Design review of the part built by this model. Coordinates are the model's own, in mm. Face numbers are marked on the shaded views. A direction names the side the tool comes from. Round coordinates to 2 decimals unless told otherwise and drop trailing zeros. Write each loop counter-clockwise with the first axis right and the second up, starting at its lowest first coordinate (ties: lowest second). Pieces come first, ordered by that corner, then holes. Notation, with made-up numbers: (15, -33.75) -> (29, -33.75) arc R24 cw to (29, -9.75) -> close; hole circle Ø5 at (76, 72.5). An arc over 180 degrees is marked (long way). Write item = value, one per line. Start each with the question number.
Item 1: Mouldability with a two-part tool opening along Z and no side actions: class the marked faces 1, 2 and 3 as released by +Z, released by -Z, zero draft, split by the parting line, or undercut.
Item 2: Add section C-C, the plane y = 0.6. State the section outline as (x, z) points.
Item 3: Add section D-D, the plane z = 1.5. State the section outline as (x, y) points.
Item 4: To check wall thickness, follow L1, parallel to Z at x = 3, y = 3.55; L2, parallel to Z at x = -2.25, y = 4; L3, parallel to X at y = 1.8, z = 4. State the ranges of each line that lie inside material, in increasing order.
Item 5: Machinability: for the marked faces 4 and 5, which of the approach directions +Z, -Z, +X, -X, +Y, -Y give a long, thin tool a straight path to every point of the face, cutting with its end or side? Answer none if there is none.
Item 6: Add section A-A, the plane x = 0. State the section outline as (y, z) points.
Item 7: For pin 1 Ø1 at (x, y) = (1.5, 3) entering from +Z; pin 2 Ø2.5 at (x, z) = (0, -4) entering from -Y; pin 3 Ø6 at (x, z) = (0, 4) entering from +Y; pin 4 Ø1 at (x, y) = (-4, 0.5) entering from -Z, all flat-tipped, find the tip position at first contact; note any pin that passes through.
Item 8: Add section B-B, the plane z = -5. State the section outline as (x, y) points, then the cut area to 3 significant figures.
from build123d import *

# Parameters (mm, degrees)
SKETCH1_R           = 7.5
SKETCH1_R_2         = 1.5
BOSS_EXTRUDE1_DEPTH = 5
SKETCH2_R           = 3.25
CUT_EXTRUDE1_DEPTH  = 1.5


with BuildPart() as part:
    # Sketch1 → Boss-Extrude1 (new body)
    with BuildSketch(Plane(origin=(0, 0, 0), x_dir=(1, 0, 0), z_dir=(0, 1, 0))):
        with Locations(Location((0, 0, 0), (0, 0, 270))):
            Circle(SKETCH1_R)
        with Locations(Location((0, 4, 0), (0, 0, 270))):
            Circle(SKETCH1_R_2, mode=Mode.SUBTRACT)
        with Locations(Location((0, -4, 0), (0, 0, 270))):
            Circle(SKETCH1_R_2, mode=Mode.SUBTRACT)
    extrude(amount=BOSS_EXTRUDE1_DEPTH)

    # Sketch2 → Cut-Extrude1 (cut)
    with BuildSketch(Plane(origin=(0, 5, 0), x_dir=(1, 0, 0), z_dir=(0, 1, 0))):
        with Locations(Location((0, 4, 0), (0, 0, 270))):
            Circle(SKETCH2_R)
        with Locations(Location((0, -4, 0), (0, 0, 270))):
            Circle(SKETCH2_R)
    extrude(amount=-CUT_EXTRUDE1_DEPTH, mode=Mode.SUBTRACT)


solid = part.part
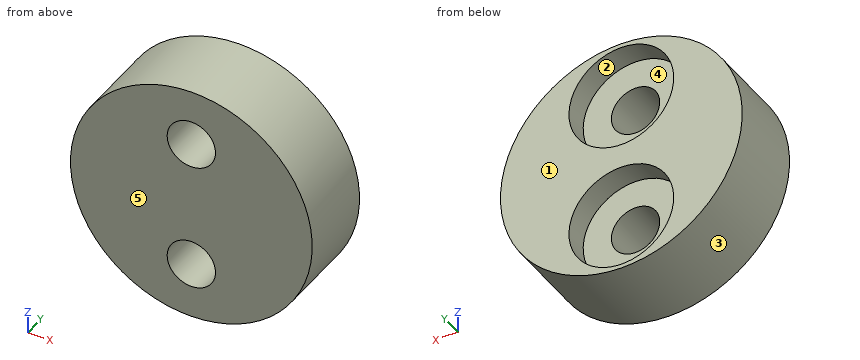
Result set:
q1.face_1 = zero draft
q1.face_2 = undercut
q1.face_3 = split by the parting line
q2.outline = circle Ø15 at (0, 0); hole circle Ø3 at (0, -4); hole circle Ø3 at (0, 4)
q3.outline = (-7.35, 0) -> (7.35, 0) -> (7.35, 5) -> (2.08, 5) -> (2.08, 3.5) -> (-2.08, 3.5) -> (-2.08, 5) -> (-7.35, 5) -> close
q4.L1 = -6.87 to -5.25, -2.75 to 2.75, 5.25 to 6.87
q4.L2 = -7.15 to -6.35, -1.65 to 1.65, 6.35 to 7.15
q4.L3 = -6.34 to -1.5, 1.5 to 6.34
q5.face_4 = +Y
q5.face_5 = +Z, -Z, +X, -X, -Y
q6.outline = (0, -7.5) -> (5, -7.5) -> (5, -7.25) -> (3.5, -7.25) -> (3.5, -5.5) -> (0, -5.5) -> close; (0, -2.5) -> (3.5, -2.5) -> (3.5, -0.75) -> (5, -0.75) -> (5, 0.75) -> (3.5, 0.75) -> (3.5, 2.5) -> (0, 2.5) -> close; (0, 5.5) -> (3.5, 5.5) -> (3.5, 7.25) -> (5, 7.25) -> (5, 7.5) -> (0, 7.5) -> close
q7.pin_1 = 7.43
q7.pin_2 = through
q7.pin_3 = 3.5
q7.pin_4 = -6.63
q8.outline = (-5.59, 0) -> (-1.12, 0) -> (-1.12, 3.5) -> (-3.09, 3.5) -> (-3.09, 5) -> (-5.59, 5) -> close; (1.12, 0) -> (5.59, 0) -> (5.59, 5) -> (3.09, 5) -> (3.09, 3.5) -> (1.12, 3.5) -> close
q8.area = 38.8 mm²
